Can you work these out from the model? Positions are in its coordinate system, mm. A direction names the side the tool comes from. Give positions to 0.01 mm unless a question says otherwise; leave off trailing zeros. Write each loop counter-clockwise with the first axis right and the second up, starting at its lowest first coordinate (ties: lowest second). Pieces come first, ordered by that corner, then holes. Notation, with made-up numbers: (6.25, 47) - (34.25, 47) arc R11 cw to (34.25, 57) - close; hole circle Ø5 at (-12.75, 72). An arc over 180 degrees is marked (long way). Use a Markdown table: item, result. Add a question column.
```python
from build123d import *

# Parameters (mm, degrees)
F1_DEPTH    = 1
F2_T        = 1
F2_T3_DEPTH = 4


# Not quite as in the source:
# - a shell that OpenCascade refuses in one call is made with other operations: the cavity is built on its own and cut out


with BuildPart() as f1:
    # F0 (on Front) → F1 (new body, symmetric)
    with BuildSketch(Plane.XZ):
        with BuildLine():
            Line((0, 29.5151724427), (0, 0))
            Line((0, 0), (3, 0))
            Line((3, 0), (3, 29.5151724427))
            ThreePointArc((3, 29.5151724427), (3.6698729811, 32.0151724427), (5.5, 33.8452994616))
            Line((5.5, 33.8452994616), (22.8205080757, 43.8452994616))
            ThreePointArc((22.8205080757, 43.8452994616), (23.7523597283, 45.059712179), (23.5525588833, 46.5773502692))
            Line((23.5525588833, 46.5773502692), (23.0525588833, 47.443375673))
            Line((23.0525588833, 47.443375673), (1.5, 35))
            Line((1.5, 35), (-20.0525588833, 47.443375673))
            Line((-20.0525588833, 47.443375673), (-20.5525588833, 46.5773502692))
            ThreePointArc((-20.5525588833, 46.5773502692), (-20.7523597283, 45.059712179), (-19.8205080757, 43.8452994616))
            Line((-19.8205080757, 43.8452994616), (-2.5, 33.8452994616))
            ThreePointArc((-2.5, 33.8452994616), (-0.6698729811, 32.0151724427), (0, 29.5151724427))
        make_face()
    extrude(amount=F1_DEPTH, both=True)

    # F2: shell of thickness 1, made by hand


with BuildPart() as f2_core1:
    # F2_t2: copy of F1
    add(f1.part)

    # the walls: a layer under each face that stays
    f2_faces = [f2_core1.faces().sort_by_distance(p)[0] for p in [
        (12.2762794416, 0, 41.2216878365),
        (23.3025588833, 0, 47.0103629711),
        (23.7523597283, 0, 45.059712179),
        (14.1602540378, 0, 38.8452994616),
        (3.6698729811, 0, 32.0151724427),
        (3, 0, 14.7575862213),
        (1.5, 0, 0),
        (0, 0, 14.7575862213),
        (-0.6698729811, 0, 32.0151724427),
        (-11.1602540378, 0, 38.8452994616),
        (-20.7523597283, 0, 45.059712179),
        (-20.3025588833, 0, 47.0103629711),
        (-9.2762794416, 0, 41.2216878365),
        (1.5, 1, 23.7216878365),
    ]]
    thicken(f2_faces, amount=-F2_T, mode=Mode.SUBTRACT)

    # F2_s4 → F2_t3 (cut)
    with BuildSketch(Plane.XZ.offset(-2)):
        Polygon((1.5, 35.0173205081), (2, 34.1339745962), (1.5, 33.8452994616), (1, 34.1339745962), align=None)
    extrude(amount=F2_T3_DEPTH, mode=Mode.SUBTRACT)


with BuildPart() as f1_1:
    add(f1.part)

    # what is left inside the walls is the cavity
    f2_cavity = [f2_core1.part.solids().sort_by_distance(p)[0] for p in [
        (1.5, -0.01, 16.025783),
    ]]
    add(f2_cavity, mode=Mode.SUBTRACT)


solid = f1_1.part
```
Q1. If we mould it in two halves opening along Z, with no side actions, what happens to faces 6 (the flat face through (13.54, -0.51, 39.64)), 7 (the cylindrical face through (-0.69, -0.01, 32.05)), 8 (the cylindrical face through (23.747, -0.014, 45.039))? For each: released by +Z, released by -Z, zero draft, split by the parting line, or undercut.
Q2. Suppose I cut it at B-B (z = 3). Please give me the cut outline in (x, y), and give its area (3 significant figures).
Q3. I'm going to push flat-ended pins straight in: P1, Ø1.1, axis at y = -0.5, z = 12.5, coming from the +X side; P2, Ø0.8, axis at y = -0.5, z = 16.5, coming from the -X side; P3, Ø0.5, axis at x = 1.5, y = -0.5, coming from the +Z side; P4, Ø12, axis at x = -3.5, z = 29.5, coming from the -Y side. Where does each tip first touch, or does it pass through?
Q4. If I drill on probe 1 along X at (y, z) = (-0.6, 44); probe 2 along X at (y, z) = (-0.6, 10.5); probe 3 along X at (y, z) = (0.8, 11.5), over which ranges is the centre line in solid material (lowest first)? Write a range as [from, to].
Q5. On a 3-axis mill with a long thin cutter (end or side, diameter ignored), from which of +Z, -Z, +X, -X, +Y, -Y can I reach the whole of each face in a straight line? I mean faces 1 (the flat face through (1.4, 0, 28.7)), 2 (the flat face through (12.43, -0.01, 41.31)), 3 (the flat face through (0, 0, 15)), 4 (the cylindrical face through (3.65, -0.01, 31.98)), 5 (the cylindrical face through (-20.758, -0.014, 45.081)). Say none if no direction works.
Q6. Suppose I cut it at A-A (y = -0.35). Please give me the cut outline in (x, z).
Q7. Suppose I cut it at C-C (z = 36.5). Please give me the cut outline in (x, y), and give its area (3 significant figures).
Q8. Suppose I cut it at D-D (x = -14). Please give me the cut outline in (y, z).
Derived:
| question | item | result |
|---|---|---|
| 1 | face 6 | undercut |
| 1 | face 7 | released by -Z |
| 1 | face 8 | split by the parting line |
| 2 | outline | (0, -1) - (1, -1) - (1, 0) - (2, 0) - (2, -1) - (3, -1) - (3, 1) - (0, 1) - close |
| 2 | area | 5.00 mm² |
| 3 | P1 | x = 3 |
| 3 | P2 | x = 0 |
| 3 | P3 | z = 35.14 |
| 3 | P4 | y = -1 |
| 4 | probe 1 | [-20.05, -18.09], [-16.09, -14.09], [17.09, 19.09], [21.09, 23.05] |
| 4 | probe 2 | [0, 1], [2, 3] |
| 4 | probe 3 | [0, 3] |
| 5 | face 1 | -Y |
| 5 | face 2 | +Z, +Y, -Y |
| 5 | face 3 | -Z, -X, +Y, -Y |
| 5 | face 4 | -Z, +X, +Y, -Y |
| 5 | face 5 | -X, +Y, -Y |
| 6 | outline | (-20.55, 46.58) arc R2 ccw to (-19.82, 43.85) - (-2.5, 33.85) arc R5 cw to (0, 29.52) - (0, 0) - (3, 0) - (3, 29.52) arc R5 cw to (5.5, 33.85) - (22.82, 43.85) arc R2 ccw to (23.55, 46.58) - (23.05, 47.44) - (1.5, 35) - (-20.05, 47.44) - close; hole (-19.69, 46.08) arc R1 ccw to (-19.32, 44.71) - (-2, 34.71) arc R6 cw to (1, 29.52) - (1, 1) - (2, 1) - (2, 29.52) arc R6 cw to (5, 34.71) - (22.32, 44.71) arc R1 ccw to (22.69, 46.08) - (1.5, 33.85) - close |
| 7 | outline | (-7.1, -1) - (-5.1, -1) - (-5.1, 0) - (-3.1, 0) - (-3.1, -1) - (-1.1, -1) - (-1.1, 1) - (-7.1, 1) - close; (4.1, -1) - (6.1, -1) - (6.1, 0) - (8.1, 0) - (8.1, -1) - (10.1, -1) - (10.1, 1) - (4.1, 1) - close |
| 7 | area | 20.0 mm² |
| 8 | outline | (-1, 40.48) - (1, 40.48) - (1, 43.95) - (-1, 43.95) - (-1, 42.79) - (0, 42.79) - (0, 41.64) - (-1, 41.64) - close |
